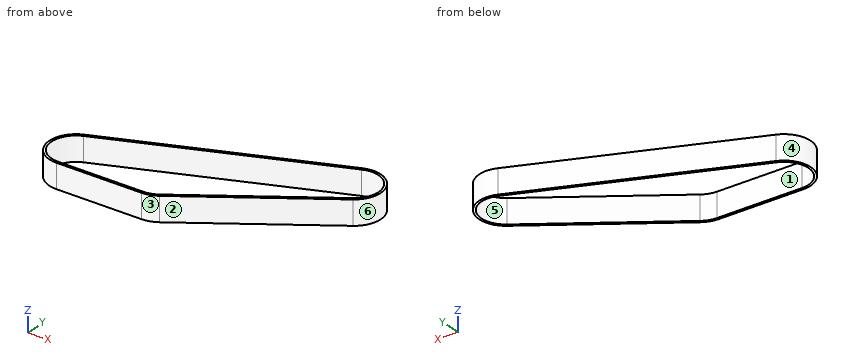
```python
from build123d import *

# Parameters (mm, degrees)
EXTRUDE_1_DEPTH = 50


with BuildPart() as part:
    # 스케치2 → 보스-돌출1 (new body)
    with BuildSketch(Plane.XY):
        with BuildLine():
            Line((-241.197082179, -39.036417247), (199.923978611, 140.464504767))
            ThreePointArc((199.923978611, 140.464504767), (268.871700929, 115.515016226), (251.177460246, 44.358995835))
            Line((251.177460246, 44.358995835), (-14.943600544, -135.14192618))
            ThreePointArc((-14.943600544, -135.14192618), (-29.552594818, -142.110059006), (-45.560530395, -144.502461007))
            Line((-45.560530395, -144.502461007), (-220.560530395, -144.502461007))
            ThreePointArc((-220.560530395, -144.502461007), (-274.293559474, -100.264408412), (-241.197082179, -39.036417247))
        make_face()
        with BuildLine():
            Line((-220.560530395, -139.750461007), (-45.560530395, -139.750461007))
            ThreePointArc((-45.560530395, -139.750461007), (-30.941945159, -137.565698805), (-17.600885222, -131.202339635))
            Line((-17.600885222, -131.202339635), (248.520175569, 48.298582379))
            ThreePointArc((248.520175569, 48.298582379), (264.678709214, 113.278875694), (201.715052802, 136.062964441))
            Line((201.715052802, 136.062964441), (-239.406007988, -43.437957574))
            ThreePointArc((-239.406007988, -43.437957574), (-269.629997336, -99.351888722), (-220.560530395, -139.750461007))
        make_face(mode=Mode.SUBTRACT)
    extrude(amount=EXTRUDE_1_DEPTH)


solid = part.part
```
Input: part model. Units: mm. Frame: model coordinates. Face numbers are marked on the shaded views. A direction names the side the tool comes from. Coordinates: 2 decimals unless noted, no trailing zeros. Write each loop counter-clockwise with the first axis right and the second up, starting at its lowest first coordinate (ties: lowest second). Pieces come first, ordered by that corner, then holes. Notation, with made-up numbers: (88, -32.75) - (99, -32.75) arc R11 ccw to (99, -28.75) - close; hole circle Ø7 at (27, -28). An arc over 180 degrees is marked (long way). Put each result on its own line as item: value. Start each with the question number.
1) Mould query, pull axis X, two halves, no side actions, for the marked faces 3, 4, 5 and 6. Classes: pulls with the +X half, pulls with the -X half, needs draft (parallel to the pull), parting line crosses it, or undercut.
2) Cut plane B-B (y = -63.5). Return the cut outline in (x, z), plus the area to 3 significant figures.
3) Contact query for flat-ended pins moving along their axis: pin 1 (5 mm diameter, centred on x = 21, z = 17, fed in from +Y); pin 2 (1 mm diameter, centred on y = 98, z = 10, fed in from +X); pin 3 (25 mm diameter, centred on x = -175.5, z = 21.5, fed in from +Y). Output: stop coordinate, or through.
4) Cut plane C-C (z = 28). Return the cut outline in (x, y).
5) Reachability of the marked faces 1 and 2 from +Z, -Z, +X, -X, +Y, -Y: full face, straight path, thin tool, end or side. Return the list, or none.
6) Ray query, L1, parallel to X at y = -54, z = 9.5; L2, parallel to Y at x = -1, z = 24.5; L3, parallel to Y at x = -74, z = 27.5. Return the intervals inside material, ascending.
7) Cut plane A-A (x = 214.5). Return the cut outline in (y, z), plus the area to 3 significant figures.
Resolved:
1. face 3: pulls with the +X half
1. face 4: pulls with the -X half
1. face 5: undercut
1. face 6: parting line crosses it
2. outline: (-268.61, 0) - (-263.12, 0) - (-263.12, 50) - (-268.61, 50) - close; (82.77, 0) - (91.27, 0) - (91.27, 50) - (82.77, 50) - close
2. area: 700 mm2
3. pin 1: stops at y = 68.67
3. pin 2: stops at x = 274.76
3. pin 3: stops at y = -7.22
4. outline: (-241.2, -39.04) arc R54.75 ccw to (-220.56, -144.5) - (-45.56, -144.5) arc R54.75 ccw to (-14.94, -135.14) - (251.18, 44.36) arc R54.75 ccw to (199.92, 140.46) - close; hole (-239.41, -43.44) arc R50 ccw to (-220.56, -139.75) - (-45.56, -139.75) arc R50 ccw to (-17.6, -131.2) - (248.52, 48.3) arc R50 ccw to (201.72, 136.06) - close
5. face 1: +Z, -Z
5. face 2: +Z, -Z, +X, -Y
6. L1: x = -262.03 to -255.52, 96.86 to 105.35
6. L2: y = -125.74 to -120, 53.57 to 58.7
6. L3: y = -144.5 to -139.75, 23.87 to 29
7. outline: (19.62, 0) - (25.35, 0) - (25.35, 50) - (19.62, 50) - close; (139.38, 0) - (144.17, 0) - (144.17, 50) - (139.38, 50) - close
7. area: 526 mm2
